Job drawing, mm, ordinate dimensions from the low corner. One solid piece. A direction names the side the tool comes from. Give positions to 0.01 mm unless a question says otherwise; leave off trailing zeros. Loops run counter-clockwise (first coordinate to the right, second up) from the corner with the lowest first, then second, coordinate; pieces in that order, holes last.
Item 1: Saw through at D-D on y = 75. Give the cut face in (x, z).
Item 2: Drop flat-ended pins along their axis: P1, Ø5, axis at x = 57.5, z = 71, coming from the -Y side; P2, Ø5, axis at x = 63.5, y = 65, coming from the -Z side; P3, Ø2, axis at x = 38, z = 68.5, coming from the +Y side; P4, Ø1, axis at x = 123.5, z = 38.5, coming from the -Y side. Give the stop position or say it passes through.
Item 3: Saw through at C-C on z = 11. Give the cut face in (x, y), plus the area to 3 significant figures.
Item 4: Saw through at B-B on x = 66.5. Give the cut face in (y, z).
Item 5: Which spindle directions (+Z, -Z, +X, -X, +Y, -Y) get a long thin tool onto all of the face, cutting with end or side? Do the marked faces 1, 2 and 3. Say none if no direction does.
Item 6: Saw through at A-A on y = 93.5. Give the cut face in (x, z), plus the area to 3 significant figures.
Item 7: Probe probe 1 along Z at (x, y) = (121, 39); probe 2 along Z at (x, y) = (166, 42); probe 3 along X at (y, z) = (5, 22). List the from-to ranges inside material, lowest first.
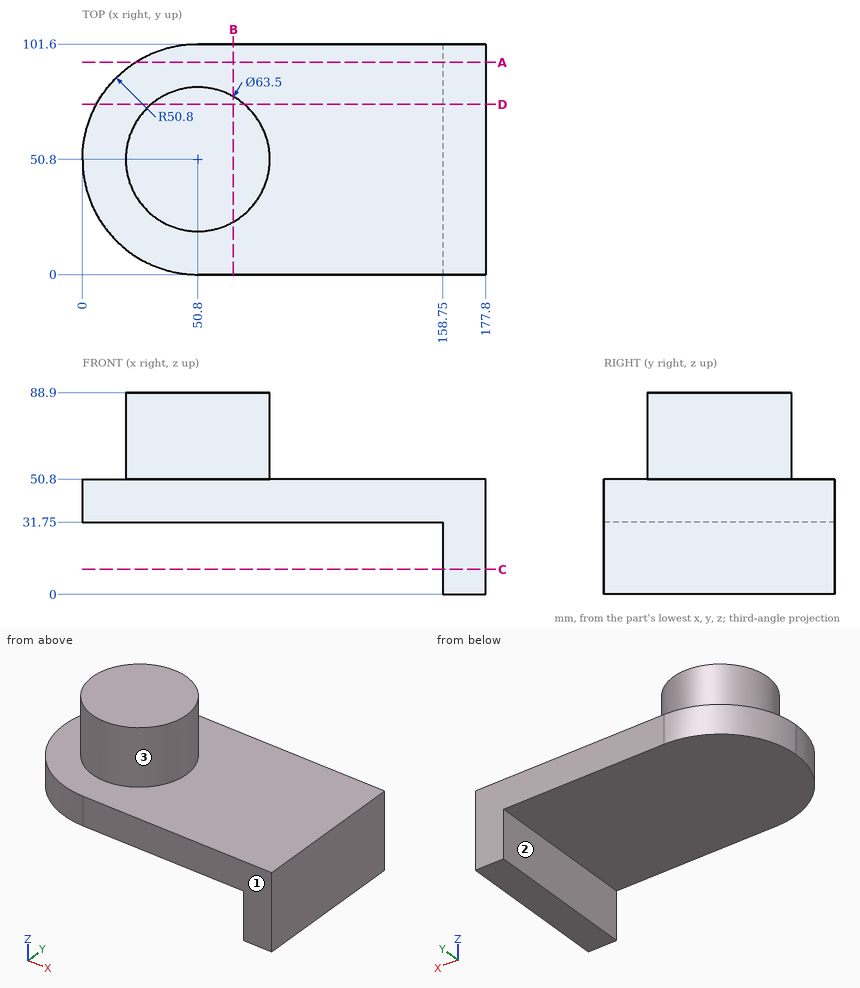
Results below:
1. outline: (6.13, 31.75) - (158.75, 31.75) - (158.75, 0) - (177.8, 0) - (177.8, 50.8) - (71.35, 50.8) - (71.35, 88.9) - (30.25, 88.9) - (30.25, 50.8) - (6.13, 50.8) - close
2. P1: stops at y = 19.33
2. P2: stops at z = 31.75
2. P3: stops at y = 80.28
2. P4: stops at y = 0
3. outline: (158.75, 0) - (177.8, 0) - (177.8, 101.6) - (158.75, 101.6) - close
3. area: 1,940 mm2
4. outline: (0, 31.75) - (101.6, 31.75) - (101.6, 50.8) - (78.4, 50.8) - (78.4, 88.9) - (23.2, 88.9) - (23.2, 50.8) - (0, 50.8) - close
5. face 1: +Z, -Z, +X, -X, -Y
5. face 2: -Z, -X, +Y, -Y
5. face 3: +Z
6. outline: (23.28, 31.75) - (158.75, 31.75) - (158.75, 0) - (177.8, 0) - (177.8, 50.8) - (23.28, 50.8) - close
6. area: 3,550 mm2
7. probe 1: z = 31.75 to 50.8
7. probe 2: z = 0 to 50.8
7. probe 3: x = 158.75 to 177.8
